from build123d import *

# Parameters (mm, degrees)
SKETCH1_W          = 125
SKETCH1_H          = 75
BASE_FLANGE1_DEPTH = 0.7
CUT_EXTRUDE1_DEPTH = 10
FILLET1_R          = 2


# Sheet-metal steps are written as plain solids
with BuildPart() as part:
    # Sketch1 → Base-Flange1 (new body)
    with BuildSketch(Plane(origin=(0, 0, 0), x_dir=(0, 0, -1), z_dir=(1, 0, 0))):
        Rectangle(SKETCH1_W, SKETCH1_H)
    extrude(amount=-BASE_FLANGE1_DEPTH)

    # Sketch10 → Cut-Extrude1 (cut)
    with BuildSketch(Plane(origin=(0, 0, 0), x_dir=(0, 0, -1), z_dir=(1, 0, 0))):
        Polygon((35.82011331, -22.5), (-47.5, 16.967422094), (-47.5, -22.5), align=None)
        Polygon((47.5, 22.5), (-35.82011331, 22.5), (47.5, -16.967422094), align=None)
    extrude(amount=-CUT_EXTRUDE1_DEPTH, mode=Mode.SUBTRACT)

    # Fillet1
    fillet1_edges = [part.edges().sort_by_distance(p)[0] for p in [
        (-0.35, 16.967422094, 47.5),
        (-0.35, -22.5, -35.82011331),
        (-0.35, -22.5, 47.5),
        (-0.35, 22.5, 35.82011331),
        (-0.35, 22.5, -47.5),
        (-0.35, -16.967422094, -47.5),
        (-0.35, -37.5, -62.5),
        (-0.35, -37.5, 62.5),
        (-0.35, 37.5, 62.5),
        (-0.35, 37.5, -62.5),
    ]]
    fillet(fillet1_edges, radius=FILLET1_R)


solid = part.part
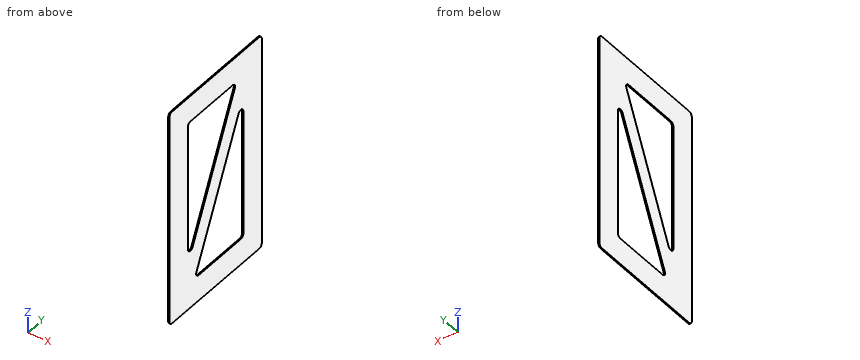
Verification items for the finished model (mm, model axes). Round coordinates to 2 decimals unless told otherwise and drop trailing zeros. Order: outer loops, then holes, each group sorted by start corner. A loop starts at its lowest first (then second) coordinate and runs counter-clockwise, first axis right, second up.
1. Thickness scan on L1, parallel to Z at x = -0.55, y = -14.5; L2, parallel to Z at x = -0.55, y = -7; L3, parallel to Y at x = -0.6, z = 20. Record the ranges inside material, lowest first.
Final values:
L1: z = -62.5 to -47.38, -42.29 to -18.93, 47.5 to 62.5
L2: z = -62.5 to -47.5, -26.46 to -3.1, 47.5 to 62.5
L3: y = -37.5 to -22.5, 3.94 to 15.01, 22.5 to 37.5
2. Section check A-A on z = -10. Record the cut outline in (x, y), then the cut area to 3 significant figures.
Final values:
outline: (-0.7, -37.5) - (0, -37.5) - (0, -22.5) - (-0.7, -22.5) - close; (-0.7, -10.27) - (0, -10.27) - (0, 0.8) - (-0.7, 0.8) - close; (-0.7, 22.5) - (0, 22.5) - (0, 37.5) - (-0.7, 37.5) - close
area: 28.7 mm2
3. Section check C-C on y = -7. Record the cut outline in (x, z).
Final values:
outline: (-0.7, -62.5) - (0, -62.5) - (0, -47.5) - (-0.7, -47.5) - close; (-0.7, -26.46) - (0, -26.46) - (0, -3.1) - (-0.7, -3.1) - close; (-0.7, 47.5) - (0, 47.5) - (0, 62.5) - (-0.7, 62.5) - close
4. Section check D-D on z = -40. Record the cut outline in (x, y).
Final values:
outline: (-0.7, -37.5) - (0, -37.5) - (0, -13.41) - (-0.7, -13.41) - close; (-0.7, 22.5) - (0, 22.5) - (0, 37.5) - (-0.7, 37.5) - close
5. Section check B-B on x = -0.3. Record the cut outline in (y, z).
Final values:
outline: (-37.5, -60.5) arc R2 ccw to (-35.5, -62.5) - (35.5, -62.5) arc R2 ccw to (37.5, -60.5) - (37.5, 60.5) arc R2 ccw to (35.5, 62.5) - (-35.5, 62.5) arc R2 ccw to (-37.5, 60.5) - close; hole (-22.5, -26.93) arc R2 ccw to (-18.69, -27.78) - (15.61, 44.64) arc R2 ccw to (13.81, 47.5) - (-20.5, 47.5) arc R2 ccw to (-22.5, 45.5) - close; hole (-15.61, -44.64) arc R2 ccw to (-13.81, -47.5) - (20.5, -47.5) arc R2 ccw to (22.5, -45.5) - (22.5, 26.93) arc R2 ccw to (18.69, 27.78) - close
